Can you work these out from the model? Positions are in its coordinate system, mm. Round coordinates to 2 decimals unless told otherwise and drop trailing zeros. Loops run counter-clockwise (first coordinate to the right, second up) from the corner with the lowest first, then second, coordinate; pieces in that order, holes last.
```python
from build123d import *

# Parameters (mm, degrees)
SKETCH_1_R               = 32
SKETCH_1_R_2             = 20
EXTRUDE_1_DEPTH          = 2
HOLE_WIZARD_M41_D        = 4.2
PATTERN_CIRCULAR_1_COUNT = 6


with BuildPart() as part:
    # Эскиз1 → Бобышка-Вытянуть1 (new body)
    with BuildSketch(Plane.XY):
        Circle(SKETCH_1_R)
        Circle(SKETCH_1_R_2, mode=Mode.SUBTRACT)
    extrude(amount=EXTRUDE_1_DEPTH)

    # Сверло под метчик  спиральное M41 (through all)
    with Locations(Plane.XY.offset(2)):
        with Locations((0, 27.5)):
            hole_wizard_m41 = Hole(HOLE_WIZARD_M41_D / 2)

    # Круговой массив1: Сверло под метчик  спиральное M41 ×6 about axis
    pattern_circular_1_axis = Axis((0, 0, 0), (0, 0, 1))
    for i in range(1, PATTERN_CIRCULAR_1_COUNT):
        add(hole_wizard_m41.rotate(pattern_circular_1_axis, i * 360 / PATTERN_CIRCULAR_1_COUNT), mode=Mode.SUBTRACT)


solid = part.part
```
(1) Suppose I cut it at A-A (x = 0). Write out the boundary of the cut face in (y, z), then the cut area to 3 significant figures.
(2) Suppose I cut it at D-D (x = 11). Write out the boundary of the cut face in (y, z).
(3) Suppose I cut it at B-B (y = 10). Write out the boundary of the cut face in (x, z), then the cut area to 3 significant figures.
(4) If I drill on line 1 (Y direction, x = 0, z = 0.7); line 2 (Y direction, x = -0.5, z = 1.5); line 3 (X direction, y = -12, z = 1.95), over which ranges is the centre line in solid material (lowest first)?
(5) For pin 1 (1 mm diameter, centred on x = 4.5, z = 2, fed in from +Y), with a flat end and sliding along its axis, tell me the tip position at first contact or that it passes through.
(6) Suppose I cut it at C-C (z = 1.35). Write out the boundary of the cut face in (x, y), then the cut area to 3 significant figures.
(7) We'd pull the mould along Y, two halves only. Please class faces 1 (the cylindrical face through (-6.94, -31.24, 0.99)), 2 (the flat face through (14, 15, 2)), 3 (the cylindrical face through (-25.82, -13.12, 0.99)), 4 (the cylindrical face through (21.813, -13.119, 0.986)): released by +Y, released by -Y, zero draft, split by the parting line, or undercut.
Check result:
1. outline: (-32, 0) - (-29.6, 0) - (-29.6, 2) - (-32, 2) - close; (-25.4, 0) - (-20, 0) - (-20, 2) - (-25.4, 2) - close; (20, 0) - (25.4, 0) - (25.4, 2) - (20, 2) - close; (29.6, 0) - (32, 0) - (32, 2) - (29.6, 2) - close
1. area: 31.2 mm2
2. outline: (-30.05, 0) - (-16.7, 0) - (-16.7, 2) - (-30.05, 2) - close; (16.7, 0) - (30.05, 0) - (30.05, 2) - (16.7, 2) - close
3. outline: (-30.4, 0) - (-17.32, 0) - (-17.32, 2) - (-30.4, 2) - close; (17.32, 0) - (30.4, 0) - (30.4, 2) - (17.32, 2) - close
3. area: 52.3 mm2
4. line 1: y = -32 to -29.6, -25.4 to -20, 20 to 25.4, 29.6 to 32
4. line 2: y = -32 to -29.54, -25.46 to -19.99, 19.99 to 25.46, 29.54 to 32
4. line 3: x = -29.66 to -24.98, -22.65 to -16, 16 to 22.65, 24.98 to 29.66
5. pin 1: stops at y = 31.75
6. outline: circle Ø64 at (0, 0); hole circle Ø4.2 at (-23.82, -13.75); hole circle Ø4.2 at (-23.82, 13.75); hole circle Ø40 at (0, 0); hole circle Ø4.2 at (0, -27.5); hole circle Ø4.2 at (0, 27.5); hole circle Ø4.2 at (23.82, -13.75); hole circle Ø4.2 at (23.82, 13.75)
6. area: 1,880 mm2
7. face 1: split by the parting line
7. face 2: zero draft
7. face 3: undercut
7. face 4: undercut
